Input: part model. Units: mm. Frame: model coordinates. A direction names the side the tool comes from. Round coordinates to 2 decimals unless told otherwise and drop trailing zeros. Loops run counter-clockwise (first coordinate to the right, second up) from the corner with the lowest first, then second, coordinate; pieces in that order, holes last.
(1) Cut plane C-C, the plane y = 22. Output: boundary loops of the cut face in (x, z).
(2) Cut plane B-B, the plane y = 14.1. Output: boundary loops of the cut face in (x, z).
(3) Cut plane A-A, the plane y = 35.5. Output: boundary loops of the cut face in (x, z), and give its area (3 significant figures).
(4) Draft query along Y for faces 5 (the face through (-2.44, 1.67, 0.54)), 6 (the face through (0.751, -0.115, -12.218)), 7 (the face through (0, 0, -3)). Return one class per face: released by +Y, released by -Y, zero draft, split by the parting line, or undercut.
(5) Line query: line 1 (X direction, y = 22.5, z = 12.5); line 2 (Y direction, x = 0, z = -14); line 3 (Z direction, x = 14, y = 21). Output: solid intervals per line, ascending.
(6) First-contact query: pin 1 Ø5 at (y, z) = (21.1, 7) entering from -X; pin 2 Ø7.5 at (x, z) = (1.5, 1) entering from +Y; pin 3 Ø7 at (y, z) = (21.1, 0) entering from +X. Flat tips, straight axial feed; report the tip coordinate or a pass-through.
(7) Cut plane D-D, the plane x = 1. Give the number of separate pieces and of enclosed holes in the cut face, and give its area (3 significant figures).
(8) Access query for faces 1 (the face through (-7.91, -7.93, 10.316)), 2 (the face through (-14.159, 26.636, -0.325)), 3 (the face through (17, 15, 0)), 4 (the face through (11.989, 5.104, 0.249)). Directions: +Z, -Z, +X, -X, +Y, -Y. A direction counts if a zero-diameter tool reaches every point of the face in a straight line with its end or side. Return the directions, or none.
from build123d import *

# Parameters (mm, degrees)
SKETCH1_W               = 34
SKETCH1_H               = 35.6
BOSS_EXTRUDE1_DEPTH     = 3.3
BOSS_EXTRUDE2_DEPTH     = 3.5
BOSS_EXTRUDE3_START     = -30.7
BOSS_EXTRUDE3_DEPTH     = 3.3
SKETCH4_R               = 2.5
SKETCH4_R_2             = 1.5
CUT_EXTRUDE1_DEPTH      = 12
SKETCH4_3_R             = 10.925
SKETCH4_3_R_2           = 1.5
SKETCH4_3_R_3           = 2.5
CUT_EXTRUDE2_DEPTH      = 2.2
SKETCH5_R               = 4
CUT_EXTRUDE3_DEPTH      = 12.2
CUT_EXTRUDE4_DEPTH      = 47.033140236
CUT_EXTRUDE4_DEPTH_BACK = 47.033140236
SKETCH6_R               = 2.5
FILLET1_R               = 6
SKETCH7_R               = 13
SKETCH7_R_2             = 11
BOSS_EXTRUDE4_DEPTH     = 15
CHAMFER1_SIZE           = 2
FILLET2_R               = 3
SKETCH9_R               = 2.5
CUT_EXTRUDE5_DEPTH      = 15


with BuildPart() as part:
    # Sketch1 → Boss-Extrude1 (new body)
    with BuildSketch(Plane(origin=(0, 0, 0), x_dir=(1, 0, 0), z_dir=(0, 1, 0))):
        Rectangle(SKETCH1_W, SKETCH1_H)
    extrude(amount=BOSS_EXTRUDE1_DEPTH)

    # Sketch3 → Boss-Extrude2 (add)
    with BuildSketch(Plane.ZY.offset(17)):
        with BuildLine():
            Line((0, 38.9), (0, 3.3))
            Line((0, 3.3), (17.8, 3.3))
            Line((17.8, 3.3), (17.8, 21.1))
            ThreePointArc((17.8, 21.1), (12.586500705, 33.686500705), (0, 38.9))
        make_face()
        with BuildLine():
            Line((-17.8, 3.3), (0, 3.3))
            Line((0, 3.3), (0, 38.9))
            ThreePointArc((0, 38.9), (-12.586500705, 33.686500705), (-17.8, 21.1))
            Line((-17.8, 21.1), (-17.8, 3.3))
        make_face()
    extrude(amount=-BOSS_EXTRUDE2_DEPTH)

    # Sketch3<4> → Boss-Extrude3 (add)
    with BuildSketch(Plane.ZY.offset(17).offset(BOSS_EXTRUDE3_START)):
        with BuildLine():
            Line((-17.8, 3.3), (0, 3.3))
            Line((0, 3.3), (0, 38.9))
            ThreePointArc((0, 38.9), (-12.586500705, 33.686500705), (-17.8, 21.1))
            Line((-17.8, 21.1), (-17.8, 3.3))
        make_face()
        with BuildLine():
            Line((0, 38.9), (0, 3.3))
            Line((0, 3.3), (17.8, 3.3))
            Line((17.8, 3.3), (17.8, 21.1))
            ThreePointArc((17.8, 21.1), (12.586500705, 33.686500705), (0, 38.9))
        make_face()
    extrude(amount=-BOSS_EXTRUDE3_DEPTH)

    # Sketch4 → Cut-Extrude1 (cut)
    with BuildSketch(Plane.ZY.offset(17)):
        with Locations((0, 21.1)):
            Circle(SKETCH4_R)
        with Locations((7, 21.1)):
            Circle(SKETCH4_R_2)
        with Locations((0, 28.1)):
            Circle(SKETCH4_R_2)
        with Locations((-7, 21.1)):
            Circle(SKETCH4_R_2)
        with Locations((0, 14.1)):
            Circle(SKETCH4_R_2)
    extrude(amount=-CUT_EXTRUDE1_DEPTH, mode=Mode.SUBTRACT)

    # Sketch4<3> → Cut-Extrude2 (cut)
    with BuildSketch(Plane.ZY.offset(17)):
        with Locations((0, 21.1)):
            Circle(SKETCH4_3_R)
        with Locations((0, 28.1)):
            Circle(SKETCH4_3_R_2, mode=Mode.SUBTRACT)
        with Locations((0, 14.1)):
            Circle(SKETCH4_3_R_2, mode=Mode.SUBTRACT)
        with Locations((-7, 21.1)):
            Circle(SKETCH4_3_R_2, mode=Mode.SUBTRACT)
        with Locations((7, 21.1)):
            Circle(SKETCH4_3_R_2, mode=Mode.SUBTRACT)
        with Locations((0, 21.1)):
            Circle(SKETCH4_3_R_3, mode=Mode.SUBTRACT)
    extrude(amount=-CUT_EXTRUDE2_DEPTH, mode=Mode.SUBTRACT)

    # Sketch5 → Cut-Extrude3 (cut)
    with BuildSketch(Plane(origin=(17, 0, 0), x_dir=(0, 0, -1), z_dir=(1, 0, 0))):
        with Locations((0, 21.1)):
            Circle(SKETCH5_R)
    extrude(amount=-CUT_EXTRUDE3_DEPTH, mode=Mode.SUBTRACT)

    # Sketch6 → Cut-Extrude4 (cut, two sides: drawn at the far end of the back side and taken through both)
    with BuildSketch(Plane.XZ.offset(-CUT_EXTRUDE4_DEPTH_BACK)):
        with Locations(Location((0, 0, 0), (0, 0, 270))):
            Circle(SKETCH6_R)
    extrude(amount=CUT_EXTRUDE4_DEPTH + CUT_EXTRUDE4_DEPTH_BACK, mode=Mode.SUBTRACT)

    # Fillet1
    fillet1_edges = [part.edges().sort_by_distance(p)[0] for p in [
        (-13.5, 3.3, 0),
        (13.7, 3.3, 0),
    ]]
    fillet(fillet1_edges, radius=FILLET1_R)

    # Sketch7 → Boss-Extrude4 (add)
    with BuildSketch(Plane.XZ):
        with Locations(Location((0, 0, 0), (0, 0, 270))):
            Circle(SKETCH7_R)
        with Locations(Location((0, 0, 0), (0, 0, 270))):
            Circle(SKETCH7_R_2, mode=Mode.SUBTRACT)
    extrude(amount=BOSS_EXTRUDE4_DEPTH)

    # Chamfer1
    chamfer1_edges = [part.edges().sort_by_distance(p)[0] for p in [
        (0, -15, 13),
    ]]
    chamfer(chamfer1_edges, length=CHAMFER1_SIZE - 0.0001)  # a hair under: the kernel refuses the full size

    # Fillet2
    fillet2_edges = [part.edges().sort_by_distance(p)[0] for p in [
        (0, 0, 13),
    ]]
    fillet(fillet2_edges, radius=FILLET2_R)

    # Sketch9 → Cut-Extrude5 (cut)
    with BuildSketch(Plane(origin=(0, 0, -17.8), x_dir=(-1, 0, 0), z_dir=(0, 0, -1))):
        with Locations(Location((0, -2.5, 0), (0, 0, 90))):
            Circle(SKETCH9_R)
    extrude(amount=-CUT_EXTRUDE5_DEPTH, mode=Mode.SUBTRACT)


solid = part.part
Reported:
1. outline: (-17, -17.78) - (-13.5, -17.78) - (-13.5, -8.2) - (-14.8, -8.2) - (-14.8, -10.89) - (-17, -10.89) - close; (-17, 10.89) - (-14.8, 10.89) - (-14.8, 8.2) - (-13.5, 8.2) - (-13.5, 17.78) - (-17, 17.78) - close; (-14.8, -5.8) - (-13.5, -5.8) - (-13.5, -2.33) - (-14.8, -2.33) - close; (-14.8, 2.33) - (-13.5, 2.33) - (-13.5, 5.8) - (-14.8, 5.8) - close; (13.7, -17.78) - (17, -17.78) - (17, -3.9) - (13.7, -3.9) - close; (13.7, 3.9) - (17, 3.9) - (17, 17.78) - (13.7, 17.78) - close
2. outline: (-17, -17.8) - (-13.5, -17.8) - (-13.5, -1.5) - (-14.8, -1.5) - (-14.8, -8.39) - (-17, -8.39) - close; (-17, 8.39) - (-14.8, 8.39) - (-14.8, 1.5) - (-13.5, 1.5) - (-13.5, 17.8) - (-17, 17.8) - close; (13.7, -17.8) - (17, -17.8) - (17, 17.8) - (13.7, 17.8) - close
3. outline: (-17, -10.46) - (-13.5, -10.46) - (-13.5, 10.46) - (-17, 10.46) - close; (13.7, -10.46) - (17, -10.46) - (17, 10.46) - (13.7, 10.46) - close
3. area: 142 mm2
4. face 5: zero draft
4. face 6: undercut
4. face 7: released by -Y
5. line 1: x = -17 to -13.5, 13.7 to 17
5. line 2: y = 0 to 3.3
5. line 3: z = -17.8 to -4, 4 to 17.8
6. pin 1: stops at x = -14.8
6. pin 2: stops at y = 3.3
6. pin 3: stops at x = -13.5
7. separate pieces: 3
7. enclosed holes: 0
7. area: 152 mm2
8. face 1: -Y
8. face 2: -X
8. face 3: +Z, -Z, +X, +Y, -Y
8. face 4: +Z, -Z, +Y
